Geometry check sheet. Reference: the model listing, model coordinates, mm. Face numbers are marked on the shaded views. A direction names the side the tool comes from. Round coordinates to 2 decimals unless told otherwise and drop trailing zeros. Write each loop counter-clockwise with the first axis right and the second up, starting at its lowest first coordinate (ties: lowest second). Pieces come first, ordered by that corner, then holes. Notation, with made-up numbers: M 72,88 L 128,88 A20 cw 128,126 Z; hole C 58.25,-23 d11. An arc over 180 degrees is marked long. Use a Markdown table: item, result.
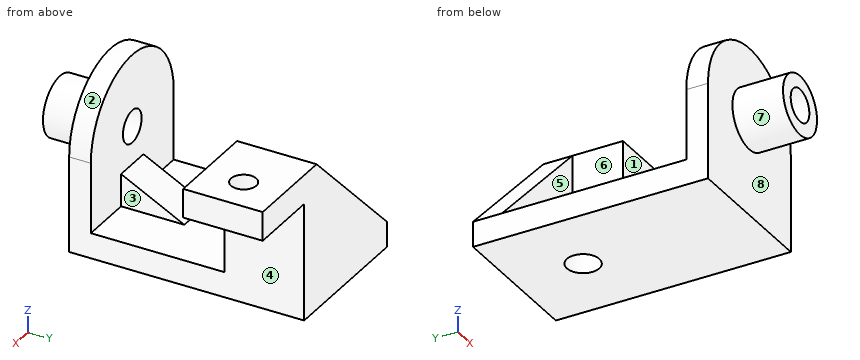
```python
from build123d import *

# Parameters (mm, degrees)
CROQUIS1_W              = 20
CROQUIS1_H              = 13.25
SALIENTE_EXTRUIR1_DEPTH = 3
CROQUIS3_R              = 2.25
CORTAR_EXTRUIR1_DEPTH   = 3
CROQUIS7_W              = 20
CROQUIS7_H              = 3.5
SALIENTE_EXTRUIR4_DEPTH = 25
CROQUIS6_R              = 4.1
CROQUIS6_R_2            = 2.25
SALIENTE_EXTRUIR3_DEPTH = 7
CROQUIS8_R              = 2.25
CORTAR_EXTRUIR3_DEPTH   = 23
NERVIO6_REACH           = 37.527
CROQUIS20_WALL_W        = 82.892721144
CROQUIS20_WALL_H        = 5.4
CROQUIS28_W             = 20
CROQUIS28_H             = 4.5
SALIENTE_EXTRUIR6_DEPTH = 3.5
CROQUIS29_W             = 3
CROQUIS29_H             = 11
SALIENTE_EXTRUIR7_DEPTH = 16.75
CROQUIS31_W             = 4
CROQUIS31_H             = 11
SALIENTE_EXTRUIR8_DEPTH = 10
CROQUIS27_R             = 1.75
CORTAR_EXTRUIR5_DEPTH   = 24
NERVIO7_REACH           = 49.84
CROQUIS32_WALL_W        = 121.545885618
CROQUIS32_WALL_H        = 4


with BuildPart() as part:
    # Croquis1 → Saliente-Extruir1 (new body)
    with BuildSketch(Plane(origin=(0, 0, 0), x_dir=(1, 0, 0), z_dir=(0, 1, 0))):
        with Locations((-8.715974267, 12.820975022)):
            Rectangle(CROQUIS1_W, CROQUIS1_H)
        with BuildLine():
            Line((-18.715974267, 6.195975022), (1.284025733, 6.195975022))
            ThreePointArc((1.284025733, 6.195975022), (-8.715974267, -3.804024978), (-18.715974267, 6.195975022))
        make_face()
    extrude(amount=SALIENTE_EXTRUIR1_DEPTH)

    # Croquis3 → Cortar-Extruir1 (cut)
    with BuildSketch(Plane(origin=(0, 3, 0), x_dir=(1, 0, 0), z_dir=(0, 1, 0))):
        with Locations(Location((-8.715974267, 6.195975022, 0), (0, 0, 270))):
            Circle(CROQUIS3_R)
    extrude(amount=-CORTAR_EXTRUIR1_DEPTH, mode=Mode.SUBTRACT)

    # Croquis7 → Saliente-Extruir4 (add)
    with BuildSketch(Plane(origin=(0, 3, 0), x_dir=(1, 0, 0), z_dir=(0, 1, 0))):
        with Locations((-8.715974267, 17.695975022)):
            Rectangle(CROQUIS7_W, CROQUIS7_H)
    extrude(amount=SALIENTE_EXTRUIR4_DEPTH)

    # Croquis6 → Saliente-Extruir3 (add)
    with BuildSketch(Plane.XZ):
        with Locations(Location((-8.715974267, -6.195975022, 0), (0, 0, 90))):
            Circle(CROQUIS6_R)
        with Locations(Location((-8.715974267, -6.195975022, 0), (0, 0, 90))):
            Circle(CROQUIS6_R_2, mode=Mode.SUBTRACT)
    extrude(amount=SALIENTE_EXTRUIR3_DEPTH)

    # Croquis8 → Cortar-Extruir3 (cut)
    with BuildSketch(Plane(origin=(0, 0, -19.445975022), x_dir=(-1, 0, 0), z_dir=(0, 0, -1))):
        with Locations((8.715974267, 23)):
            Circle(CROQUIS8_R)
    extrude(amount=-CORTAR_EXTRUIR3_DEPTH, mode=Mode.SUBTRACT)

    # Croquis20 wall → Nervio6 (add, up to next)
    with BuildSketch(Plane(origin=(-8.715974267, 7.375, -13.695975022), x_dir=(0, -0.889287802318, 0.457348012621), z_dir=(0, 0.457348012621, 0.889287802318)), mode=Mode.PRIVATE) as nervio6_sk1:
        Rectangle(CROQUIS20_WALL_W, CROQUIS20_WALL_H)
    nervio6_tool1 = extrude(nervio6_sk1.sketch, amount=-NERVIO6_REACH, mode=Mode.PRIVATE) - part.part
    add(nervio6_tool1.solids().sort_by_distance((-8.715974267, 7.375, -13.695975022))[0])

    # Croquis28 → Saliente-Extruir6 (add)
    with BuildSketch(Plane.XY.offset(-15.945975022)):
        with Locations((-8.715974267, 30.25)):
            Rectangle(CROQUIS28_W, CROQUIS28_H)
    extrude(amount=-SALIENTE_EXTRUIR6_DEPTH)

    # Croquis29 → Saliente-Extruir7 (add)
    with BuildSketch(Plane.XY.offset(-15.945975022)):
        with Locations((-0.215974267, 27)):
            Rectangle(CROQUIS29_W, CROQUIS29_H)
    extrude(amount=SALIENTE_EXTRUIR7_DEPTH)

    # Croquis31 → Saliente-Extruir8 (add)
    with BuildSketch(Plane(origin=(1.284025733, 0, 0), x_dir=(0, 0, -1), z_dir=(1, 0, 0))):
        with Locations((1.195975022, 27)):
            Rectangle(CROQUIS31_W, CROQUIS31_H)
    extrude(amount=SALIENTE_EXTRUIR8_DEPTH)

    # Croquis27 → Cortar-Extruir5 (cut)
    with BuildSketch(Plane.XY.offset(-15.945975022)):
        with Locations(Location((6.284025733, 27, 0), (0, 0, 180))):
            Circle(CROQUIS27_R)
    extrude(amount=CORTAR_EXTRUIR5_DEPTH, mode=Mode.SUBTRACT)

    # Croquis32 wall → Nervio7 (add, up to next)
    with BuildSketch(Plane(origin=(-10.215974267, 32.5, -7.570975022), x_dir=(-0.712325066938, 0, -0.701849698306), z_dir=(-0.701849698306, 0, 0.712325066938)), mode=Mode.PRIVATE) as nervio7_sk1:
        with Locations((0, 2)):
            Rectangle(CROQUIS32_WALL_W, CROQUIS32_WALL_H)
    nervio7_tool1 = extrude(nervio7_sk1.sketch, amount=-NERVIO7_REACH, mode=Mode.PRIVATE) - part.part
    add(nervio7_tool1.solids().sort_by_distance((-10.215974267, 32.5, -7.570975022))[0])


solid = part.part
```
Item 1: Mould release check, pull along Y, two halves, no side actions. Record for the marked faces 6, 7 and 8: +Y half, -Y half, draft (parallel to the pull), parting line (faces both ways), or undercut.
Outcome:
| item | result |
|---|---|
| face 6 | undercut |
| face 7 | draft |
| face 8 | -Y half |
Item 2: Cross-section at B-B, the plane z = 0. Record the cut outline in (x, y), and give its area (3 significant figures).
Outcome:
| item | result |
|---|---|
| outline | M -16.57,0 L -0.87,0 L -0.87,3 L -16.57,3 Z; M -2.53,28.5 L -1.72,28.5 L -1.72,21.5 L 11.28,21.5 L 11.28,32.5 L -2.53,32.5 Z; hole C 6.28,27 d3.5 |
| area | 184 mm2 |
Item 3: Cross-section at A-A, the plane y = 23. Record the cut outline in (x, z).
Outcome:
| item | result |
|---|---|
| outline | M -18.72,-19.45 L -10.97,-19.45 L -10.97,-15.95 L -18.72,-15.95 Z; M -6.47,-19.45 L 1.28,-19.45 L 1.28,-3.2 L 11.28,-3.2 L 11.28,0.8 L -1.72,0.8 L -1.72,-15.95 L -6.47,-15.95 Z |
Item 4: Go/stop test with flat-tipped pins: pin 1 (7 mm diameter, centred on x = -8.72, y = 23, fed in from +Z); pin 2 (2 mm diameter, centred on y = 23.5, z = -10, fed in from -X); pin 3 (5.5 mm diameter, centred on x = 6, y = 26, fed in from +Z); pin 4 (8 mm diameter, centred on y = 7.5, z = -5, fed in from +X). Record where each tip stops, or that it passes through.
Outcome:
| item | result |
|---|---|
| pin 1 | stops at z = -15.95 |
| pin 2 | stops at x = -1.72 |
| pin 3 | stops at z = 0.8 |
| pin 4 | passes through |
Item 5: Cross-section at D-D, the plane z = -9. Record the cut outline in (x, y).
Outcome:
| item | result |
|---|---|
| outline | M -18.72,0 L -11.71,0 L -11.71,-7 L -5.72,-7 L -5.72,0 L 1.28,0 L 1.28,3 L -18.72,3 Z; M -11.67,28.5 L -1.72,28.5 L -1.72,21.5 L 1.28,21.5 L 1.28,32.5 L -11.67,32.5 Z |
Item 6: Material ranges on line 1 along Y through (x, z) = (-2, 0); line 2 along Y through (x, z) = (-16, -11.5); line 3 along Y through (x, z) = (-8, -9), recorded low to high. Write a range as from..to.
Outcome:
| item | result |
|---|---|
| line 1 | y = 0..3, 28.5..32.5 |
| line 2 | y = 0..3 |
| line 3 | y = -7..3, 28.5..32.5 |
Item 7: Cross-section at C-C, the plane y = 27. Record the cut outline in (x, z), and give its area (3 significant figures).
Outcome:
| item | result |
|---|---|
| outline | M -18.72,-19.45 L 1.28,-19.45 L 1.28,-3.2 L 4.53,-3.2 L 4.53,0.8 L -1.72,0.8 L -1.72,-15.95 L -18.72,-15.95 Z; M 8.03,-3.2 L 11.28,-3.2 L 11.28,0.8 L 8.03,0.8 Z |
| area | 146 mm2 |
Item 8: Access from +Z, -Z, +X, -X, +Y, -Y to the whole of each face (thin tool, end or side, straight path). Record for the marked faces 1, 2, 3, 4 and 5.
Outcome:
| item | result |
|---|---|
| face 1 | +Z, +X, -X |
| face 2 | +Z, -Y |
| face 3 | +Z, +X |
| face 4 | -Z, +X, +Y, -Y |
| face 5 | +Z, -X |
